Autodesk Inventor part; units mm, degrees
ref_plane "YZ Plane" through (0, 0, 0) normal (1, 0, 0) x (0, 1, 0)
ref_plane "XZ Plane" through (0, 0, 0) normal (0, 1, 0) x (-1, 0, 0)
ref_plane "XY Plane" through (0, 0, 0) normal (0, 0, 1) x (1, 0, 0)
sketch "Sketch1" plane through (0, 0, 0) normal (1, 0, 0) x (0, 1, 0)
  line L0 (-6, 6) -> (6, 6)
  line L1 (6, 6) -> (6, -6)
  line L2 (6, -6) -> (-6, -6)
  line L3 (-6, -6) -> (-6, 6)
  line L4 (-6, 6) -> (6, -6) construction
  line L5 (6, 6) -> (-6, -6) construction
  point P0 (0, 0)
  dimension "d0" = 12
  dimension "d1" = 12
extrude "Extrusion1" add sketch "Sketch1" along normal blind 20
sketch "Sketch2" plane through (0, -6, 6) normal (0, 0, 1) x (1, 0, 0)
  line L0 (0, 0) -> (0, 12)
  line L1 (0, 12) -> (-6.9282, 0)
  line L2 (0, 12) -> (15.674, 12) construction
  line L3 (0, 0) -> (-6.9282, 0)
  line L4 (0, 0) -> (20, 0)
  line L5 (0, 0) -> (0, 12)
  point P0 (0, 6)
  dimension "d4" = 120
extrude "Extrusion2" add sketch "Sketch2" against normal blind 12
sketch "Sketch3" plane through (20, 0, 0) normal (1, 0, 0) x (0, 0, -1)
  circle A0 centre (0, 0) radius 4
  dimension "d7" = 8
extrude "Extrusion3" add sketch "Sketch3" along normal blind 14
sketch "Sketch4" plane through (20, 6, 6) normal (0, 1, 0) x (1, 0, 0)
  circle A0 centre (-10, 6) radius 2.5
  line L0 (-20, 0) -> (-20, 12)
  line L1 (-20, 0) -> (0, 0)
  point P0 (-20, 6)
  dimension "d10" = 5
  dimension "d11" = 10
  dimension "d12" = 6
extrude "Extrusion4" add sketch "Sketch4" along normal blind 3.75
sketch "Sketch5" plane through (20, -6, 6) normal (0, 0, 1) x (1, 0, 0)
  line L0 (0, 0) -> (-26.9282, 0)
  line L1 (-26.9282, 0) -> (-24.9282, 0)
  line L2 (-24.9282, 0) -> (-24.9282, 3.4641)
  line L3 (-26.9282, 0) -> (-20, 12)
  line L4 (-26.9282, 0) -> (-24.9282, 3.4641)
  point P0 (-20, 6)
  dimension "d15" = 2
extrude "Extrusion5" cut sketch "Sketch5" against normal blind 12
sketch "Sketch6" plane through (-4.9282, -6, 6) normal (-1, 0, 0) x (0, 0, 1)
  line L0 (0, 0) -> (-12, 0)
  line L1 (0, 0) -> (-2.5, 0)
  line L2 (-2.5, 0) -> (-2.5, 12)
  line L3 (-12, 12) -> (0, 12)
  line L4 (-2.5, 12) -> (0, 12)
  line L5 (0, 12) -> (0, 0)
  line L6 (-12, 0) -> (-12, 3.4641)
  line L7 (-12, 0) -> (-9.5, 0)
  line L8 (-9.5, 0) -> (-9.5, 12)
  line L9 (-9.5, 12) -> (-12, 12)
  line L10 (-12, 3.4641) -> (-12, 12)
  line L11 (-12, 12) -> (-12, 0)
  point P0 (-6, 6)
  dimension "d18" = 2.5
  dimension "d19" = 2.5
extrude "Extrusion6" cut sketch "Sketch6" against normal blind 4.5 contours L0 L2 L3 L5 | L0 L6 L10 L3 L8
fillet "Fillet1" radius 2 4 edges at (-0.4282, -0.3708, 3.5) (-0.4282, -0.3708, -3.5) (-0.4282, -0.3708, -6) (-0.4282, -0.3708, 6)
sketch "Sketch7" plane through (20, -6, 6) normal (0, 0, 1) x (1, 0, 0)
  line L0 (-20, 12) -> (-18.7201, 12)
  line L1 (-20, 12) -> (-16, 12)
  line L2 (-20.5742, 11.0055) -> (-22.4282, 7.7942)
  line L3 (-16, 12) -> (-22.4282, 7.7942)
  line L4 (-22.4282, 7.7942) -> (-20, 12)
  point P0 (-20, 6)
  dimension "d23" = 4
extrude "Extrusion7" cut sketch "Sketch7" against normal blind 20
sketch "Sketch8" plane through (20, -6, 6) normal (0, 0, 1) x (1, 0, 0)
  line L0 (-16, 12) -> (-18.7201, 10.2203)
  line L1 (-24.9282, 3.4641) -> (-22.4282, 7.7942)
  line L2 (-16, 12) -> (-24.9282, 3.4641)
  line L3 (-24.9282, 3.4641) -> (-24.9282, 12)
  line L4 (-16, 12) -> (0, 12)
  line L5 (-24.9282, 12) -> (-16, 12)
  point P0 (-20, 6)
extrude "Extrusion8" cut sketch "Sketch8" against normal blind 20
properties part number "18 pin schieter"
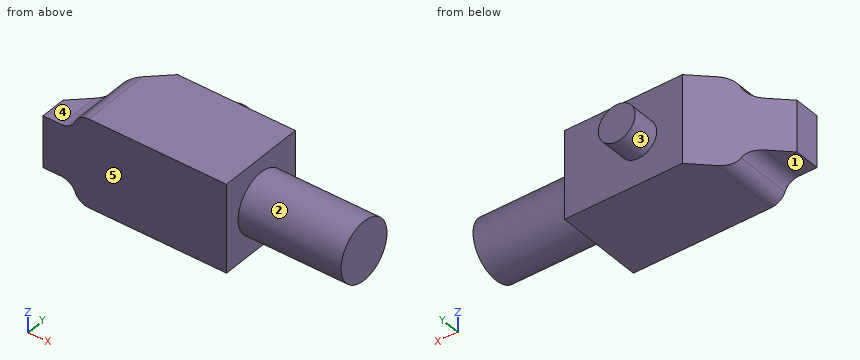
Read the model definition and answer for the solid it produces. Units are mm, in the model's axes. Face numbers are marked on the shaded views. A direction names the side the tool comes from. Round coordinates to 2 decimals unless told otherwise and drop trailing zeros. Loops run counter-clockwise (first coordinate to the right, second up) from the corner with the lowest first, then second, coordinate; pieces in that order, holes last.
Q1. Consider probe 1 along Y at (x, z) = (24, 0); probe 2 along Y at (x, z) = (13.5, 0); probe 3 along Z at (x, y) = (-3, -1.75). Determine where each line is inside the solid, lowest interval first.
Q2. Section D-D on x = 26 is taken. Write down the section's boundary in (y, z).
Q3. Section C-C on y = 2.25 is taken. Write down the section's boundary in (x, z), and give its area (3 significant figures).
Q4. Each of these flat-tipped pins is pushed along its axis until it touches: pin 1 (1 mm diameter, centred on y = 2, z = 2, fed in from -X); pin 2 (6 mm diameter, centred on x = 2.5, z = -0.5, fed in from +Y); pin 3 (2 mm diameter, centred on x = -4, y = -4, fed in from +Z); pin 4 (1.5 mm diameter, centred on x = 22.5, y = 6, fed in from +Z). Where does it stop, or does it pass through?
Q5. Which of the six approach directions +Z, -Z, +X, -X, +Y, -Y give full straight-line access (tool end or side, diameter ignored) to the marked faces 1, 2, 3, 4 and 5?
Q6. Section B-B on x = 10 is taken. Write down the section's boundary in (y, z).
Q7. Section A-A on z = 0 is taken. Write down the section's boundary in (x, y), and give its area (3 significant figures).
Output:
1. probe 1: y = -4 to 4
1. probe 2: y = -6 to 6
1. probe 3: z = -3.5 to 3.5
2. outline: circle Ø8 at (0, 0)
3. outline: (0.08, -5.6) arc R2 ccw to (1.28, -6) - (20, -6) - (20, -3.31) - (34, -3.31) - (34, 3.31) - (20, 3.31) - (20, 6) - (1.28, 6) arc R2 ccw to (0.08, 5.6) - close
3. area: 331 mm2
4. pin 1: stops at x = -0.71
4. pin 2: stops at y = 6
4. pin 3: stops at z = 3.5
4. pin 4: passes through
5. face 1: -Z, -X, +Y, -Y
5. face 2: +X
5. face 3: +Y
5. face 4: +Z, -X, +Y, -Y
5. face 5: +Z, -Z, +X, -X, -Y
6. outline: (-6, -6) - (6, -6) - (6, -2.5) - (9.75, -2.5) - (9.75, 2.5) - (6, 2.5) - (6, 6) - (-6, 6) - close
7. outline: (-4.93, -6) - (20, -6) - (20, -4) - (34, -4) - (34, 4) - (20, 4) - (20, 6) - (12.5, 6) - (12.5, 9.75) - (7.5, 9.75) - (7.5, 6) - (4, 6) - (-4.93, -2.54) - close
7. area: 392 mm2
